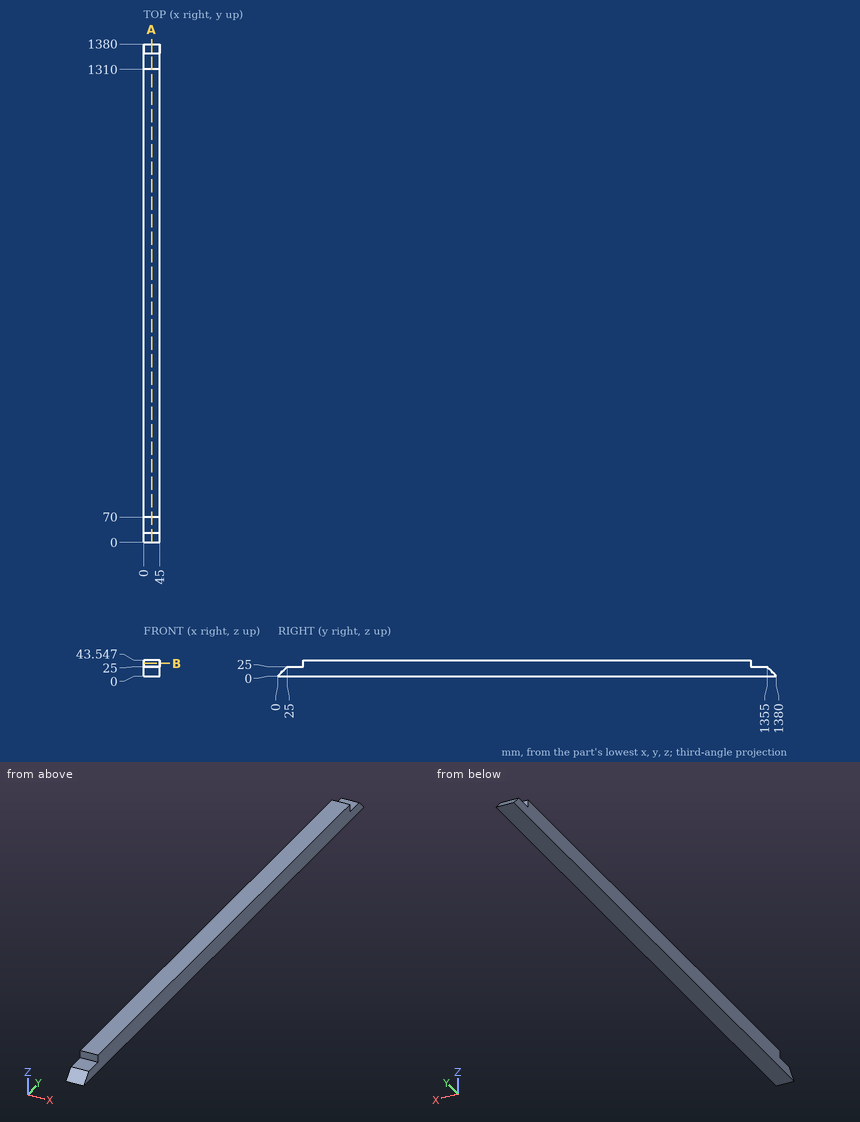
Job drawing, mm, ordinate dimensions from the low corner. One solid piece. Round coordinates to 2 decimals unless told otherwise and drop trailing zeros. Order: outer loops, then holes, each group sorted by start corner. A loop starts at its lowest first (then second) coordinate and runs counter-clockwise, first axis right, second up. Notation, with made-up numbers: (42, 62.5) - (96, 62.5) arc R30 cw to (96, 86.5) - close; hole circle Ø2 at (4.25, 3.5). An arc over 180 degrees is marked (long way). Use CSV: the item, a comma, the result in double quotes. Start each with the question number.
1) Pin check, flat tips, straight feed: pin 1 Ø13.5 at (x, y) = (25.5, 1337) entering from +Z; pin 2 Ø15 at (x, z) = (27.5, 36) entering from -Y; pin 3 Ø4 at (x, z) = (35.5, 20.5) entering from +Y. Stop position of each tip, or through.
2) Wall check: L1, parallel to Y at x = 36, z = 38.5; L2, parallel to Y at x = 36.5, z = 13.5. Give the ranges that are in metal, low to high. Write a range as [from, to].
3) Saw through at B-B (z = 35). List the corners of the cut face in (x, y).
4) Saw through at A-A (x = 21.5). List the corners of the cut face in (y, z).
Values follow:
1,pin 1,"stops at z = 25"
1,pin 2,"stops at y = 70"
1,pin 3,"stops at y = 1361.5"
2,L1,"y = [70, 1310]"
2,L2,"y = [13.5, 1366.5]"
3,outline,"(0, 70) - (45, 70) - (45, 1310) - (0, 1310) - close"
4,outline,"(0, 0) - (1380, 0) - (1355, 25) - (1310, 25) - (1310, 43.55) - (70, 43.55) - (70, 25) - (25, 25) - close"
